Autodesk Fusion 360 part; units mm, degrees
sketch "Sketch1" plane through (0, 0, 0) normal (0, 0, 1) x (1, 0, 0)
  line L0 (0, 0) -> (171.45, 0)
  line L1 (171.45, 0) -> (171.45, 76.2)
  line L2 (171.45, 76.2) -> (0, 76.2)
  line L3 (0, 76.2) -> (0, 0)
  line L4 (-19.05, -19.05) -> (190.5, -19.05)
  line L5 (190.5, -19.05) -> (190.5, 95.25)
  line L6 (190.5, 95.25) -> (-19.05, 95.25)
  line L7 (-19.05, 95.25) -> (-19.05, -19.05)
  line L8 (0, 76.2) -> (-19.05, 76.2)
  line L9 (-19.05, 76.2) -> (171.45, 76.2)
  line L10 (171.45, 76.2) -> (190.5, 76.2)
  line L11 (186.5, 91.25) -> (-15.05, 91.25)
  line L12 (-15.05, 91.25) -> (-15.05, -15.05)
  line L13 (-15.05, -15.05) -> (186.5, -15.05)
  line L14 (186.5, -15.05) -> (186.5, 91.25)
  line L15 (0, 38.1) -> (-6, 38.1) construction
  line L16 (171.45, 38.1) -> (177.45, 38.1) construction
  circle A0 centre (-6, 38.1) radius 1.5
  circle A1 centre (177.45, 38.1) radius 1.5
  line L17 (85.725, 0) -> (85.725, -6) construction
  circle A2 centre (85.725, -6) radius 1.5
  dimension "d1" = 171.45
  dimension "d2" = 76.2
  dimension "d3" = 19.05
  dimension "d4" = -4
  dimension "d15" = 6
  dimension "d16" = 6
  dimension "d17" = 3
  dimension "d18" = 3
  dimension "d19" = 6
  dimension "d20" = 3
extrude "Extrude1" add sketch "Sketch1" against normal blind 76.2 contours L0 L1 L3 L8 L9 L10 L12 L13 L14 | L4 L5 L7 L8 L9 L10 L12 L13 L14 | A0 | A1 | A2
extrude "Extrude2" add sketch "Sketch1" along normal blind 4 from surface at -76.2 contours L0 L1 L2 L3 L9 | L0 L1 L3 L8 L9 L10 L12 L13 L14 | L4 L5 L7 L8 L9 L10 L12 L13 L14 | A0 | A1 | A2
extrude "Extrude3" cut sketch "Sketch1" along normal blind 68 from surface at -72.2 contours L0 L1 L3 L8 L9 L10 L12 L13 L14 | A0 | A1 | A2
fillet "Fillet1" radius 15 13 edges at (-15.05, 30.575, -72.2) (85.725, -15.05, -72.2) (-15.05, -15.05, -38.2) (-15.05, 30.575, -4.2) (85.725, -15.05, -4.2) (186.5, 30.575, -4.2) (186.5, 30.575, -72.2) (186.5, -15.05, -38.2) (-19.05, -19.05, -38.1) (-19.05, 28.575, -76.2) (85.725, -19.05, -76.2) (190.5, 28.575, -76.2) (190.5, -19.05, -38.1)
extrude "Extrude4" cut sketch "Sketch1" against normal blind 20 contours A0 | A1 | A2
Work out the finished part from the listing and answer in its coordinate system (mm). A direction names the side the tool comes from. Coordinates: 2 decimals unless noted, no trailing zeros. Write each loop counter-clockwise with the first axis right and the second up, starting at its lowest first coordinate (ties: lowest second). Pieces come first, ordered by that corner, then holes.
1. For a pull along X with two mould halves and no side action, classify faces 1 (the cylindrical face through (186.22, 36.64, -71.69)), 2 (the flat face through (84, -3, 0)), 3 (the cylindrical face through (-10.77, -10.54, -37.93)) as +X half, -X half, draft (parallel to the pull), parting line (faces both ways), or undercut.
Results list:
face 1: +X half
face 2: draft
face 3: undercut
2. The part is cut by section B-B, the plane x = 74. Write down the section's boundary in (y, z).
Results list:
outline: (-19.05, -61.2) arc R15 ccw to (-4.05, -76.2) - (76.2, -76.2) - (76.2, -72.2) - (-0.05, -72.2) arc R15 cw to (-15.05, -57.2) - (-15.05, -19.2) arc R15 cw to (-0.05, -4.2) - (0, -4.2) - (0, 0) - (-19.05, 0) - close
3. Flat-ended cylindrical pins translate along their axes: pin 1 (2.5 mm diameter, centred on x = 85.725, y = -6, fed in from -Z); pin 2 (2.5 mm diameter, centred on x = 177.45, y = 38.1, fed in from +Z); pin 3 (3 mm diameter, centred on x = 106, z = -47.5, fed in from +Y). Find the tip coordinate at first contact, or state that the pin passes through.
Results list:
pin 1: stops at z = -76.18
pin 2: stops at z = -70.36
pin 3: stops at y = -15.05
4. The part is cut by section A-A, the plane y = 16. Write down the section's boundary in (x, z), and give its area (3 significant figures).
Results list:
outline: (-19.05, -61.2) arc R15 ccw to (-4.05, -76.2) - (175.5, -76.2) arc R15 ccw to (190.5, -61.2) - (190.5, 0) - (171.45, 0) - (171.45, -4.2) - (171.5, -4.2) arc R15 cw to (186.5, -19.2) - (186.5, -57.2) arc R15 cw to (171.5, -72.2) - (-0.05, -72.2) arc R15 cw to (-15.05, -57.2) - (-15.05, -19.2) arc R15 cw to (-0.05, -4.2) - (0, -4.2) - (0, 0) - (-19.05, 0) - close
area: 1,640 mm2
5. The part is cut by section D-D, the plane z = -17. Write down the section's boundary in (x, y), and give its area (3 significant figures).
Results list:
outline: (-19.05, -4.05) arc R15 ccw to (-4.05, -19.05) - (175.5, -19.05) arc R15 ccw to (190.5, -4.05) - (190.5, 76.2) - (186.34, 76.2) - (186.34, -0.05) arc R14.84 cw to (171.5, -14.89) - (-0.05, -14.89) arc R14.84 cw to (-14.89, -0.05) - (-14.89, 76.2) - (-19.05, 76.2) - close
area: 1,630 mm2
6. Consider line 1 along X through (y, z) = (38.1, -3); line 2 along X through (y, z) = (25.5, -52.5); line 3 along Z through (x, y) = (140, 28). Determine where each line is inside the solid, lowest interval first.
Results list:
line 1: x = -19.05 to -7.5, -4.5 to 0, 171.45 to 175.95, 178.95 to 190.5
line 2: x = -19.05 to -15.05, 186.5 to 190.5
line 3: z = -76.2 to -72.2
7. For faces 4 (the flat face through (85, 0, -2)), 5 (the flat face through (84, 37, -76.2)), 6 (the cylindrical face through (86.93, -10.77, -67.69)), determine the directions among +Z, -Z, +X, -X, +Y, -Y from which every point of the face is accessible in a straight line to the end or side of a thin tool.
Results list:
face 4: +Z, +Y
face 5: -Z, +X, -X, +Y, -Y
face 6: +Y
8. The part is cut by section C-C, the plane z = -44.5. Write down the section's boundary in (x, y), and give its area (3 significant figures).
Results list:
outline: (-19.05, -4.05) arc R15 ccw to (-4.05, -19.05) - (175.5, -19.05) arc R15 ccw to (190.5, -4.05) - (190.5, 76.2) - (186.5, 76.2) - (186.5, -0.05) arc R15 cw to (171.5, -15.05) - (-0.05, -15.05) arc R15 cw to (-15.05, -0.05) - (-15.05, 76.2) - (-19.05, 76.2) - close
area: 1,570 mm2
